Geometry check sheet. Reference: the model listing, model coordinates, mm. A direction names the side the tool comes from. Round coordinates to 2 decimals unless told otherwise and drop trailing zeros. Order: outer loops, then holes, each group sorted by start corner. A loop starts at its lowest first (then second) coordinate and runs counter-clockwise, first axis right, second up.
(1) Set-up check for faces 1 (the face through (-23, -9, -16.354)), 2 (the face through (-206.22, -9.39, 0.81)), 3 (the face through (-23, -9, 16.354)): record each of +Z, -Z, +X, -X, +Y, -Y from which the full face is reachable in a straight line by a thin tool's end or side.
(2) Sectioned sample at B-B (y = -6.75). Record the boundary of the cut face in (x, z), plus the area to 3 significant figures.
(3) Sectioned sample at C-C (x = -129.5). Record the boundary of the cut face in (y, z), plus the area to 3 significant figures.
(4) Material ranges on line 1 along Z through (x, y) = (-142, -5); line 2 along X through (y, z) = (-15, -17); line 3 along X through (y, z) = (-9.25, -19.5), recorded low to high.
(5) Go/stop test with flat-tipped pins: pin 1 (4 mm diameter, centred on x = -32, y = -15.5, fed in from -Z); pin 2 (10 mm diameter, centred on y = -10, z = -19.5, fed in from -X); pin 3 (4.5 mm diameter, centred on y = -11.5, z = 19, fed in from +X). Record where each tip stops, or that it passes through.
(6) Sectioned sample at A-A (z = -19.5). Record the boundary of the cut face in (x, y), plus the area to 3 significant figures.
from build123d import *

# Parameters (mm, degrees)
F0_W     = 362.554728
F0_H     = 32.70875
F1_R     = 24.119355
F1_W     = 59.741348
F1_H     = 50.58742
F2_DEPTH = 19.05


with BuildPart() as f2:
    # F0 (on Front) + F1 (on face) → F2 (new body)
    with BuildSketch(Plane.XZ):
        Rectangle(F0_W, F0_H)
    with BuildSketch(Plane.XZ):
        with Locations((-182.114676, 0)):
            Circle(F1_R)
        with Locations((151.280463, 0)):
            Rectangle(F1_W, F1_H)
    extrude(amount=F2_DEPTH)

    # F3: union 


solid = f2.part
Answer below:
1. face 1: -Z, +Y, -Y
1. face 2: +Y, -Y
1. face 3: +Z, +Y, -Y
2. outline: (-164.39, -16.35) - (121.41, -16.35) - (121.41, -25.29) - (181.15, -25.29) - (181.15, -16.35) - (181.28, -16.35) - (181.28, 16.35) - (181.15, 16.35) - (181.15, 25.29) - (121.41, 25.29) - (121.41, 16.35) - (-164.39, 16.35) arc R24.12 ccw (long way) to start
2. area: 14,100 mm2
3. outline: (-19.05, -16.35) - (0, -16.35) - (0, 16.35) - (-19.05, 16.35) - close
3. area: 623 mm2
4. line 1: z = -16.35 to 16.35
4. line 2: x = -199.22 to -165, 121.41 to 181.15
4. line 3: x = -196.31 to -167.92, 121.41 to 181.15
5. pin 1: stops at z = -16.35
5. pin 2: stops at x = -201.39
5. pin 3: stops at x = 181.15
6. outline: (-196.31, -19.05) - (-167.92, -19.05) - (-167.92, 0) - (-196.31, 0) - close; (121.41, -19.05) - (181.15, -19.05) - (181.15, 0) - (121.41, 0) - close
6. area: 1,680 mm2
